Source: CAD feature listing. Evaluate the final solid. Frame: model axes, mm. Face numbers are marked on the shaded views. A direction names the side the tool comes from. Round coordinates to 2 decimals unless told otherwise and drop trailing zeros. Loops run counter-clockwise (first coordinate to the right, second up) from the corner with the lowest first, then second, coordinate; pieces in that order, holes last. Notation, with made-up numbers: M 69,52 L 110,52 A7 cw 110,65 Z; hole C 31.25,12 d4. An arc over 180 degrees is marked long. Write each question's results on one line, items separated by ' | '. Start each with the question number.
1. Section B-B on y = 87.5. Give the number of separate pieces and of enclosed holes in the cut face, and give its area (3 significant figures).
2. Section A-A on z = -8.5. Output: boundary loops of the cut face in (x, y).
3. Ray query, line 1 (X direction, y = 31, z = -9.5); line 2 (X direction, y = 80.5, z = -8.5); line 3 (Y direction, x = -33, z = -5.75). Return the intervals inside material, ascending.
4. Set-up query: the marked faces 3 and 4. Return all of +Z, -Z, +X, -X, +Y, -Y with unobstructed straight access to the full face (end or side cutting, diameter ignored); none if empty.
5. Draft query along Y for the marked faces 1 and 2. Return one class per face: released by +Y, released by -Y, zero draft, split by the parting line, or undercut.
6. Contact query for flat-ended pins moving along their axis: pin 1 Ø4 at (x, z) = (6, -4.5) entering from +Y; pin 2 Ø6 at (x, z) = (-21.5, -8) entering from +Y; pin 3 Ø2 at (x, z) = (-38, -9) entering from -Y; pin 4 Ø12 at (x, y) = (5, 70.5) entering from -Z. Output: stop coordinate, or through.
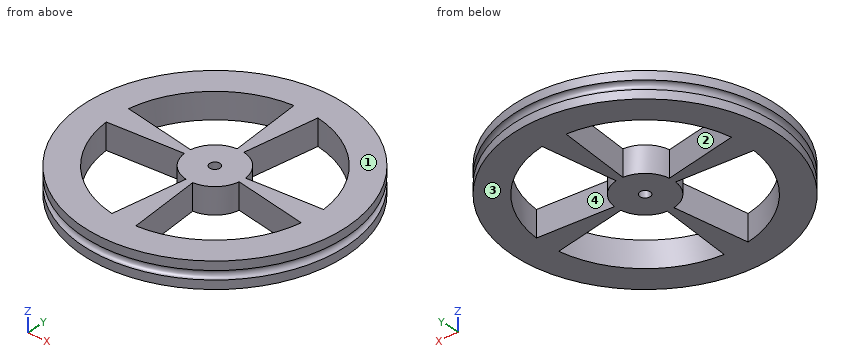
from build123d import *

# Parameters (mm, degrees)
SKETCH5_R          = 2.1
CUT_EXTRUDE1_DEPTH = 120.743736371
CUT_EXTRUDE2_DEPTH = 120.743736371


with BuildPart() as part:
    # Sketch3 → Revolve1 (revolve)
    with BuildSketch(Plane(origin=(0, 0, 0), x_dir=(0, 0, -1), z_dir=(1, 0, 0))):
        with BuildLine():
            Line((0, 0), (0, 53.34))
            Line((0, 53.34), (10.62, 53.34))
            Line((10.62, 53.34), (10.62, 0))
            Line((10.62, 0), (7.08, 0))
            ThreePointArc((7.08, 0), (5.3147, 1.7653), (3.5494, 0))
            Line((3.5494, 0), (0, 0))
        make_face()
    revolve(axis=Axis((0, 53.34, 0), (0, 0, -1)))

    # Sketch5 → Cut-Extrude1 (cut, through all)
    with BuildSketch(Plane.XY):
        with Locations((0, 53.34)):
            Circle(SKETCH5_R)
    extrude(amount=-CUT_EXTRUDE1_DEPTH, mode=Mode.SUBTRACT)

    # Sketch6 → Cut-Extrude2 (cut, through all)
    with BuildSketch(Plane.XY):
        with BuildLine():
            Line((6.358903838, 94.508420539), (1.788715657, 64.920391883))
            ThreePointArc((1.788715657, 64.920391883), (8.538481175, 61.364918635), (11.668962152, 54.407849322))
            Line((11.668962152, 54.407849322), (41.483288818, 57.136216085))
            ThreePointArc((41.483288818, 57.136216085), (30.354394508, 81.868674027), (6.358903838, 94.508420539))
        make_face()
        with BuildLine():
            Line((41.168420539, 46.981096162), (11.580391883, 51.551284343))
            ThreePointArc((11.580391883, 51.551284343), (8.024918635, 44.801518825), (1.067849322, 41.671037848))
            Line((1.067849322, 41.671037848), (3.796216085, 11.856711182))
            ThreePointArc((3.796216085, 11.856711182), (28.528674027, 22.985605492), (41.168420539, 46.981096162))
        make_face()
        with BuildLine():
            Line((-6.358903838, 12.171579461), (-1.788715657, 41.759608117))
            ThreePointArc((-1.788715657, 41.759608117), (-8.538481175, 45.315081365), (-11.668962152, 52.272150678))
            Line((-11.668962152, 52.272150678), (-41.483288818, 49.543783915))
            ThreePointArc((-41.483288818, 49.543783915), (-30.354394508, 24.811325973), (-6.358903838, 12.171579461))
        make_face()
        with BuildLine():
            Line((-41.168420539, 59.698903838), (-11.580391883, 55.128715657))
            ThreePointArc((-11.580391883, 55.128715657), (-8.024918635, 61.878481175), (-1.067849322, 65.008962152))
            Line((-1.067849322, 65.008962152), (-3.796216085, 94.823288818))
            ThreePointArc((-3.796216085, 94.823288818), (-28.528674027, 83.694394508), (-41.168420539, 59.698903838))
        make_face()
    extrude(amount=-CUT_EXTRUDE2_DEPTH, mode=Mode.SUBTRACT)


solid = part.part
Taken from the geometry:
1) separate pieces: 3 | enclosed holes: 0 | area: 440 mm^2
2) outline: C 0,53.34 d106.68; hole M -41.48,49.54 A41.66 ccw -6.36,12.17 L -1.79,41.76 A11.72 cw -11.67,52.27 Z; hole M -41.17,59.7 L -11.58,55.13 A11.72 cw -1.07,65.01 L -3.8,94.82 A41.66 ccw Z; hole C 0,53.34 d4.2; hole M 1.07,41.67 L 3.8,11.86 A41.66 ccw 41.17,46.98 L 11.58,51.55 A11.72 cw Z; hole M 1.79,64.92 A11.72 cw 11.67,54.41 L 41.48,57.14 A41.66 ccw 6.36,94.51 Z
3) line 1: -48.44 to -35.16, -3.45 to 2.04, 35.16 to 48.44 | line 2: -45.91 to -31.58, -2.49 to 4.2, 31.58 to 45.91 | line 3: 13.63 to 27.92, 50.32 to 58.44, 78.76 to 93.05
4) face 3: -Z, +X, -X, +Y, -Y | face 4: +Z, -Z
5) face 1: zero draft | face 2: undercut
6) pin 1: y = 106.51 | pin 2: y = 103.37 | pin 3: y = 14.92 | pin 4: z = -10.62
